Drawing for the job (mm, zero at the part's lowest x, y, z). A direction names the side the tool comes from. Round coordinates to 2 decimals unless told otherwise and drop trailing zeros. Order: outer loops, then holes, each group sorted by start corner. A loop starts at its lowest first (then second) coordinate and runs counter-clockwise, first axis right, second up. Notation, with made-up numbers: M 34.5,46 L 75.5,46 A34 cw 75.5,81 Z; hole C 12.25,26.5 d9. An arc over 180 degrees is marked long. Answer as CSV lines item,"result". Start each with the question number.
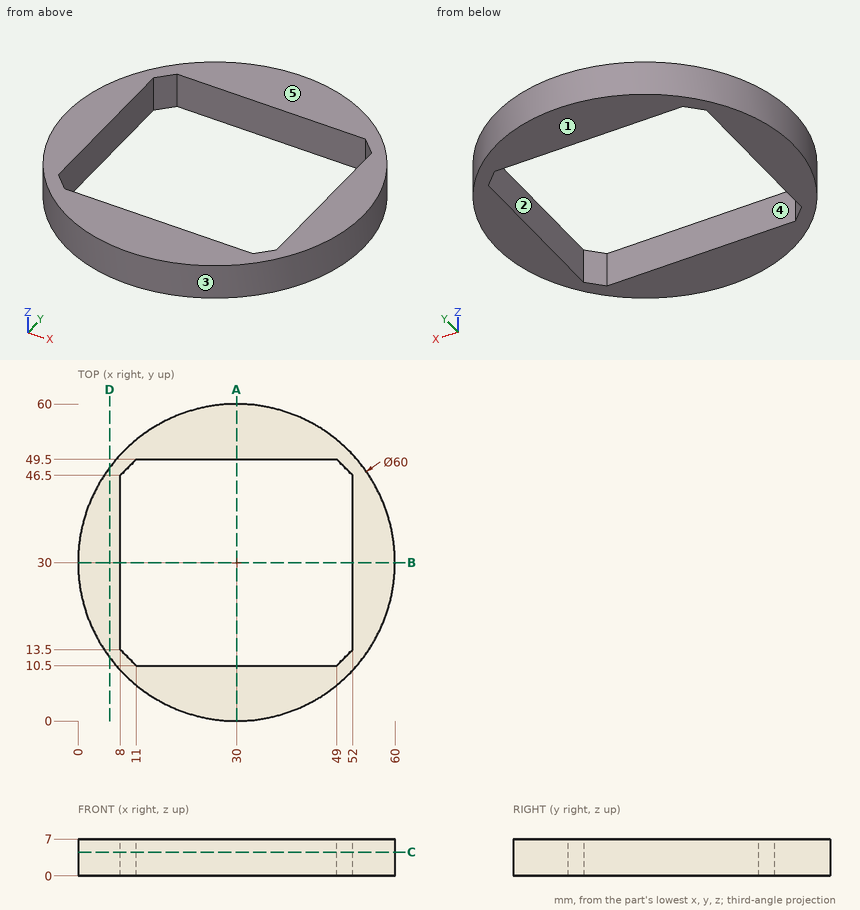
Q1. Tool access for the marked faces 4 and 5: list every direction of +Z, -Z, +X, -X, +Y, -Y with a clear straight run to the whole face (end or side of a thin tool).
Q2. Drop flat-ended pins along their axis: P1, Ø4, axis at x = 28, z = 3.5, coming from the +Y side; P2, Ø8, axis at x = 19, y = 42, coming from the -Z side; P3, Ø1.5, axis at x = 47, z = 4, coming from the -Y side; P4, Ø2, axis at y = 23, z = 3.5, coming from the +X side. Give the stop position or say it passes through.
Q3. Band-saw the part on A-A, the plane x = 30. Write the cut outline in (y, z).
Q4. Mould opens along Y. For the marked faces 1, 2 and 3 say: +Y half, -Y half, draft (parallel to the pull), parting line (faces both ways), or undercut.
Q5. Probe line 1 along Y through (x, z) = (33, 5.25); line 2 along Y through (x, z) = (31, 1.75); line 3 along X through (y, z) = (19, 6.25). List the from-to ranges inside material, lowest first. Write a range as from..to.
Q6. Band-saw the part on D-D, the plane x = 6. Write the cut outline in (y, z).
Q7. Band-saw the part on C-C, the plane z = 4.5. Write the cut outline in (x, y).
Q8. Band-saw the part on B-B, the plane y = 30. Write the cut outline in (x, z), then the cut area to 3 significant figures.
Answer:
1,face 4,"+Z, -Z"
1,face 5,"+Z, +X, -X, +Y, -Y"
2,P1,"stops at y = 60"
2,P2,"passes through"
2,P3,"stops at y = 4.78"
2,P4,"stops at x = 59.39"
3,outline,"M 0,0 L 10.5,0 L 10.5,7 L 0,7 Z; M 49.5,0 L 60,0 L 60,7 L 49.5,7 Z"
4,face 1,"draft"
4,face 2,"undercut"
4,face 3,"parting line"
5,line 1,"y = 0.15..10.5, 49.5..59.85"
5,line 2,"y = 0.02..10.5, 49.5..59.98"
5,line 3,"x = 2.09..8, 52..57.91"
6,outline,"M 12,0 L 48,0 L 48,7 L 12,7 Z"
7,outline,"C 30,30 d60; hole M 8,13.5 L 11,10.5 L 49,10.5 L 52,13.5 L 52,46.5 L 49,49.5 L 11,49.5 L 8,46.5 Z"
8,outline,"M 0,0 L 8,0 L 8,7 L 0,7 Z; M 52,0 L 60,0 L 60,7 L 52,7 Z"
8,area,"112 mm^2"
